Could you check a few things on this model? Use its own coordinates, in mm. A direction names the side the tool comes from. Round coordinates to 2 decimals unless told otherwise and drop trailing zeros. Write each loop counter-clockwise with the first axis right and the second up, starting at its lowest first coordinate (ties: lowest second). Pieces come first, ordered by that corner, then holes. Notation, with made-up numbers: (23.5, 74.5) - (31.5, 74.5) arc R18 ccw to (31.5, 98.5) - close; hole circle Ø11 at (14, 78.5). An arc over 180 degrees is marked (long way). Write each question's results on one line, items separated by ' | '. Start each with the question number.
(1) Imagine slicing it at C-C on z = 3.5. Write out the boundary of the cut face in (x, y).
(2) Imagine slicing it at A-A on y = 10. Write out the boundary of the cut face in (x, z).
(3) Imagine slicing it at B-B on x = 0. State how many separate pieces and enclosed holes the cut face has, then the cut area to 3 significant figures.
(4) For P1, Ø5, axis at x = 7.5, y = 21.5, coming from the -Z side; P2, Ø8, axis at x = -2, y = 26, coming from the +Z side; P3, Ø0.8, axis at x = -1.5, z = -0.5, coming from the -Y side; P4, Ø8, axis at y = 22, z = 16, coming from the -X side, each with a flat end and sliding along its axis, tell me the tip position at first contact or that it passes through.
(5) Imagine slicing it at D-D on y = 18. Write out the boundary of the cut face in (x, z), then the cut area to 3 significant figures.
(6) Please list where these lines run through material, in increasing order: line 1 (Y direction, x = 0, z = 3.3); line 2 (X direction, y = 20.5, z = 12); line 3 (X direction, y = 18, z = 2). Write a range as [from, to].
(7) Thinking about a two-plate mould opening in X: for faces 4 (the flat face through (8.7, 17.4, 17.1)), 5 (the flat face through (-3, 8.8, -0.5)), 6 (the flat face through (7.5, 13, 15)), which applies, +X half, -X half, draft (parallel to the pull), parting line (faces both ways), or undercut?
(8) On a 3-axis mill with a long thin cutter (end or side, diameter ignored), from which of +Z, -Z, +X, -X, +Y, -Y can I reach the whole of each face in a straight line? I mean faces 1 (the flat face through (3, -0.5, 25.5)), 2 (the flat face through (3, 11.2, -0.5)), 3 (the flat face through (1.2, 7, -0.5)). Say none if no direction works.
Autodesk Inventor part; units mm, degrees
ref_plane "bracket_to_bolt_XY" through (1, 10, 0) normal (0, 0, 1) x (1, 0, 0)
ref_plane "bracket_to_bolt_YZ" through (1, 10, 0) normal (1, 0, 0) x (0, 1, 0)
ref_plane "bracket_to_bolt_ZX" through (1, 10, 0) normal (0, 1, 0) x (0, 0, 1)
sketch "Sketch_15" plane through (0, 0, 0) normal (1, 0, 0) x (0, 1, 0)
  line L0 (0, 30) -> (0, 0)
  line L1 (0, 0) -> (30, 0)
  line L2 (30, 0) -> (30, 4.0858)
  arc A0 (30, 4.0858) -> (29.7071, 4.7929) centre (29, 4.0858) ccw
  line L3 (29.7071, 4.7929) -> (4.7929, 29.7071)
  arc A1 (4.7929, 29.7071) -> (4.0858, 30) centre (4.0858, 29) ccw
  line L4 (4.0858, 30) -> (0, 30)
extrude "Extrusion1" add sketch "Sketch_15" along normal mid plane 20
sketch "Sketch_16" plane through (0, 0, 0) normal (1, 0, 0) x (0, 1, 0)
  line L0 (2.9278, 34.5) -> (4.5, 4.5)
  line L1 (4.5, 4.5) -> (34.5, 4.5)
  line L2 (34.5, 4.5) -> (34.5, 34.5)
  line L3 (34.5, 34.5) -> (2.9278, 34.5)
extrude "Extrusion2" cut sketch "Sketch_16" along normal mid plane 15
sketch "Sketch_17" plane through (0, 4.5, 0) normal (0, 1, 0) x (1, 0, 0)
  line L0 (-5.4209, -10.5) -> (-4.4687, -18.5299)
  arc A0 (-4.4687, -18.5299) -> (4.4687, -18.5299) centre (0, -18) ccw
  line L1 (4.4687, -18.5299) -> (5.4209, -10.5)
  line L2 (5.4209, -10.5) -> (-5.4209, -10.5)
extrude "Extrusion3" add sketch "Sketch_17" against normal blind 2.25
sketch "Sketch4" plane through (10, 0, 0) normal (0, 0, -1) x (-1, 0, 0)
  point P0 (10, 18)
hole "Hole1" at (0, 18, 0) direction (0, 0, 1) diameter 5.3 depth 4.5
sketch "Sketch5" plane through (10, 0, 0) normal (0, 0, -1) x (-1, 0, 0)
  point P0 (10, 10)
hole "Hole2" at (0, 10, 0) direction (0, 0, 1) diameter 5.3 depth 4.5
sketch "Sketch6" plane through (-10, 0, 30) normal (0, -1, 0) x (1, 0, 0)
  point P0 (10, -12)
hole "Hole3" at (0, 0, 18) direction (0, 1, 0) diameter 5.3 depth 4.5
sketch "Sketch_1" plane through (0, 0, 0) normal (0, 1, 0) x (-1, 0, 0)
  line L0 (10, 0) -> (10, 30)
  line L1 (10, 30) -> (-10, 30)
  line L2 (-10, 30) -> (-10, 0)
  line L3 (-10, 0) -> (10, 0)
extrude "Extrusion4" add sketch "Sketch_1" against normal blind 1
sketch "Sketch_4" plane through (0, 0, 0) normal (0, 1, 0) x (-1, 0, 0)
  line L0 (10, 0) -> (10, 30)
  line L1 (10, 30) -> (-10, 30)
  line L2 (-10, 30) -> (-10, 0)
  line L3 (-10, 0) -> (10, 0)
  arc A0 (3, 10.7) -> (2.7, 11) centre (2.7, 10.7) ccw
  line L4 (2.7, 11) -> (-2.7, 11)
  arc A1 (-2.7, 11) -> (-3, 10.7) centre (-2.7, 10.7) ccw
  line L5 (-3, 10.7) -> (-3, 5.3)
  arc A2 (-3, 5.3) -> (-2.7, 5) centre (-2.7, 5.3) ccw
  line L6 (-2.7, 5) -> (2.7, 5)
  arc A3 (2.7, 5) -> (3, 5.3) centre (2.7, 5.3) ccw
  line L7 (3, 5.3) -> (3, 10.7)
  arc A4 (3, 26.7) -> (2.7, 27) centre (2.7, 26.7) ccw
  line L8 (2.7, 27) -> (-2.7, 27)
  arc A5 (-2.7, 27) -> (-3, 26.7) centre (-2.7, 26.7) ccw
  line L9 (-3, 26.7) -> (-3, 24.3)
  arc A6 (-3, 24.3) -> (-2.7, 24) centre (-2.7, 24.3) ccw
  line L10 (-2.7, 24) -> (2.7, 24)
  arc A7 (2.7, 24) -> (3, 24.3) centre (2.7, 24.3) ccw
  line L11 (3, 24.3) -> (3, 26.7)
extrude "Extrusion5" cut sketch "Sketch_4" against normal blind 1
sketch "Sketch_10" plane through (0, 0, 0) normal (0, 0, 1) x (1, 0, 0)
  line L0 (-10, 0) -> (10, 0)
  line L1 (10, 0) -> (10, 30)
  line L2 (10, 30) -> (-10, 30)
  line L3 (-10, 30) -> (-10, 0)
extrude "Extrusion6" add sketch "Sketch_10" against normal blind 1
sketch "Sketch_11" plane through (0, 0, 0) normal (0, 0, 1) x (1, 0, 0)
  line L0 (-10, 0) -> (10, 0)
  line L1 (10, 0) -> (10, 30)
  line L2 (10, 30) -> (-10, 30)
  line L3 (-10, 30) -> (-10, 0)
  line L4 (0.5, 7) -> (2, 7)
  arc A0 (2, 7) -> (3, 8) centre (2, 8) ccw
  line L5 (3, 8) -> (3, 9.5)
  line L6 (3, 9.5) -> (2.6024, 9.5)
  arc A1 (0.5, 7.3976) -> (2.6024, 9.5) centre (0, 10) ccw
  line L7 (0.5, 7.3976) -> (0.5, 7)
  line L8 (0.5, 13) -> (0.5, 12.6024)
  arc A2 (2.6024, 10.5) -> (0.5, 12.6024) centre (0, 10) ccw
  line L9 (2.6024, 10.5) -> (3, 10.5)
  line L10 (3, 10.5) -> (3, 12)
  arc A3 (3, 12) -> (2, 13) centre (2, 12) ccw
  line L11 (2, 13) -> (0.5, 13)
  line L12 (-3, 9.5) -> (-3, 8)
  arc A4 (-3, 8) -> (-2, 7) centre (-2, 8) ccw
  line L13 (-2, 7) -> (-0.5, 7)
  line L14 (-0.5, 7) -> (-0.5, 7.3976)
  arc A5 (-2.6024, 9.5) -> (-0.5, 7.3976) centre (0, 10) ccw
  line L15 (-2.6024, 9.5) -> (-3, 9.5)
  line L16 (-3, 10.5) -> (-2.6024, 10.5)
  arc A6 (-0.5, 12.6024) -> (-2.6024, 10.5) centre (0, 10) ccw
  line L17 (-0.5, 12.6024) -> (-0.5, 13)
  line L18 (-0.5, 13) -> (-2, 13)
  arc A7 (-2, 13) -> (-3, 12) centre (-2, 12) ccw
  line L19 (-3, 12) -> (-3, 10.5)
extrude "Extrusion7" cut sketch "Sketch_11" against normal blind 1
ref_plane "bracket_to_bolt_XY" through (1, 10, 0) normal (0, 0, 1) x (1, 0, 0)
ref_plane "bracket_to_bolt_YZ" through (1, 10, 0) normal (1, 0, 0) x (0, 1, 0)
ref_plane "bracket_to_bolt_ZX" through (1, 10, 0) normal (0, 1, 0) x (0, 0, 1)
ref_plane "bracket_to_dummy_XY" through (0, 0, 0) normal (0, 1, 0) x (1, 0, 0)
ref_plane "bracket_to_dummy_YZ" through (0, 0, 0) normal (1, 0, 0) x (0, 0, -1)
ref_plane "bracket_to_dummy_ZX" through (0, 0, 0) normal (0, 0, -1) x (0, 1, 0)
ref_plane "to_bolt_4_7_base_XY" through (0, 4.5, 18) normal (0, 1, 0) x (1, 0, 0)
ref_plane "to_bolt_4_7_base_YZ" through (0, 4.5, 18) normal (1, 0, 0) x (0, 0, -1)
ref_plane "to_bolt_4_7_base_ZX" through (0, 4.5, 18) normal (0, 0, -1) x (0, 1, 0)
ref_plane "to_bolt_row_4_to_7_XY" through (0, 18, 4.5) normal (0, 0, 1) x (1, 0, 0)
ref_plane "to_bolt_row_4_to_7_YZ" through (0, 18, 4.5) normal (1, 0, 0) x (0, 1, 0)
ref_plane "to_bolt_row_4_to_7_ZX" through (0, 18, 4.5) normal (0, 1, 0) x (0, 0, 1)
ref_plane "to_nut_base_4_7_XY" through (0, -2, 18) normal (0, 1, 0) x (1, 0, 0)
ref_plane "to_nut_base_4_7_YZ" through (0, -2, 18) normal (1, 0, 0) x (0, 0, -1)
ref_plane "to_nut_base_4_7_ZX" through (0, -2, 18) normal (0, 0, -1) x (0, 1, 0)
ref_plane "to_nut_row_4_to_7_XY" through (0, 18, -2) normal (0, 0, 1) x (1, 0, 0)
ref_plane "to_nut_row_4_to_7_YZ" through (0, 18, -2) normal (1, 0, 0) x (0, 1, 0)
ref_plane "to_nut_row_4_to_7_ZX" through (0, 18, -2) normal (0, 1, 0) x (0, 0, 1)
properties part number "HBLFSN5"
Response:
1) outline: (-10, 0) - (10, 0) - (10, 30) - (-10, 30) - close; hole circle Ø5.3 at (0, 10); hole circle Ø5.3 at (0, 18)
2) outline: (-10, 0) - (-2.65, 0) - (-2.65, 4.5) - (-7.5, 4.5) - (-7.5, 24.5) - (-10, 24.5) - close; (2.65, 0) - (10, 0) - (10, 24.5) - (7.5, 24.5) - (7.5, 4.5) - (2.65, 4.5) - close
3) separate pieces: 4 | enclosed holes: 0 | area: 178 mm²
4) P1: z = 0 | P2: z = 4.5 | P3: y = 7 | P4: x = -10
5) outline: (-10, 0) - (-2.65, 0) - (-2.65, 4.5) - (-7.5, 4.5) - (-7.5, 16.5) - (-10, 16.5) - close; (2.65, 0) - (10, 0) - (10, 16.5) - (7.5, 16.5) - (7.5, 4.5) - (2.65, 4.5) - close | area: 126 mm²
6) line 1: [0, 7.35], [12.65, 15.35], [20.65, 30] | line 2: [-10, -7.5], [7.5, 10] | line 3: [-10, -2.65], [2.65, 10]
7) face 4: draft | face 5: -X half | face 6: undercut
8) face 1: +Z, -Z, +X, -Y | face 2: -Z, +X, +Y, -Y | face 3: -Z, +X, -X, -Y
